```python
from build123d import *

# Parameters (mm, degrees)
BOSS_EXTRU_1_DEPTH      = 36
ESQUISSE2_W             = 34
ESQUISSE2_H             = 20
BOSS_EXTRU_2_DEPTH      = 2
ESQUISSE3_R             = 6
BOSS_EXTRU_3_DEPTH      = 2
ESQUISSE4_R             = 2.5
BOSS_EXTRU_4_DEPTH      = 4
ESQUISSE5_W             = 20
ESQUISSE5_H             = 2.5
BOSS_EXTRU_5_DEPTH      = 7
ENL_V_MAT_EXTRU_1_REACH = 53.585
ESQUISSE6_R             = 2
CONG_1_R                = 2
ESQUISSE7_W             = 20
ESQUISSE7_H             = 2.5
BOSS_EXTRU_6_DEPTH      = 7
ENL_V_MAT_EXTRU_2_REACH = 59.184
ESQUISSE8_R             = 2
CONG_2_R                = 2


with BuildPart() as part:
    # Esquisse1 → Boss.-Extru.1 (new body)
    with BuildSketch(Plane(origin=(0, 0, 0), x_dir=(1, 0, 0), z_dir=(0, 1, 0))):
        Polygon((0, 0), (0, 10), (40, 10), (40, -10), (0, -10), align=None)
    extrude(amount=BOSS_EXTRU_1_DEPTH)

    # Esquisse2 → Boss.-Extru.2 (add)
    with BuildSketch(Plane(origin=(0, 36, 0), x_dir=(1, 0, 0), z_dir=(0, 1, 0))):
        with Locations((23, 0)):
            Rectangle(ESQUISSE2_W, ESQUISSE2_H)
    extrude(amount=BOSS_EXTRU_2_DEPTH)

    # Esquisse3 → Boss.-Extru.3 (add)
    with BuildSketch(Plane(origin=(0, 38, 0), x_dir=(1, 0, 0), z_dir=(0, 1, 0))):
        with Locations(Location((32, 0, 0), (0, 0, 90))):
            Circle(ESQUISSE3_R)
    extrude(amount=BOSS_EXTRU_3_DEPTH)

    # Esquisse4 → Boss.-Extru.4 (add)
    with BuildSketch(Plane(origin=(0, 40, 0), x_dir=(1, 0, 0), z_dir=(0, 1, 0))):
        with Locations(Location((32, 0, 0), (0, 0, 270))):
            Circle(ESQUISSE4_R)
    extrude(amount=BOSS_EXTRU_4_DEPTH)

    # Esquisse5 → Boss.-Extru.5 (add)
    with BuildSketch(Plane.ZY):
        with Locations((0, 29.75)):
            Rectangle(ESQUISSE5_W, ESQUISSE5_H)
    extrude(amount=BOSS_EXTRU_5_DEPTH)

    # Esquisse6 → Enlèv. mat.-Extru.1 (cut, up to next)
    with BuildSketch(Plane(origin=(0, 31, 0), x_dir=(1, 0, 0), z_dir=(0, 1, 0)), mode=Mode.PRIVATE) as enl_v_mat_extru_1_sk1:
        with Locations(Location((-4.5, 5, 0), (0, 0, 270))):
            Circle(ESQUISSE6_R)
    enl_v_mat_extru_1_tool1 = extrude(enl_v_mat_extru_1_sk1.sketch, amount=-ENL_V_MAT_EXTRU_1_REACH, mode=Mode.PRIVATE) & part.part
    # Esquisse6 → Enlèv. mat.-Extru.1 (cut, up to next)
    with BuildSketch(Plane(origin=(0, 31, 0), x_dir=(1, 0, 0), z_dir=(0, 1, 0)), mode=Mode.PRIVATE) as enl_v_mat_extru_1_sk2:
        with Locations(Location((-4.5, -5, 0), (0, 0, 270))):
            Circle(ESQUISSE6_R)
    enl_v_mat_extru_1_tool2 = extrude(enl_v_mat_extru_1_sk2.sketch, amount=-ENL_V_MAT_EXTRU_1_REACH, mode=Mode.PRIVATE) & part.part
    add(enl_v_mat_extru_1_tool1.solids().sort_by_distance((-4.5, 31, -5))[0], mode=Mode.SUBTRACT)
    add(enl_v_mat_extru_1_tool2.solids().sort_by_distance((-4.5, 31, 5))[0], mode=Mode.SUBTRACT)

    # Congé1
    cong_1_edges = [part.edges().sort_by_distance(p)[0] for p in [
        (0, 14.25, 10),
        (0, 14.25, -10),
        (-7, 29.75, -10),
        (-7, 29.75, 10),
        (0, 33.5, -10),
        (0, 33.5, 10),
    ]]
    fillet(cong_1_edges, radius=CONG_1_R)

    # Esquisse7 → Boss.-Extru.6 (add)
    with BuildSketch(Plane(origin=(40, 0, 0), x_dir=(0, 0, -1), z_dir=(1, 0, 0))):
        with Locations((0, 29.75)):
            Rectangle(ESQUISSE7_W, ESQUISSE7_H)
    extrude(amount=BOSS_EXTRU_6_DEPTH)

    # Esquisse8 → Enlèv. mat.-Extru.2 (cut, up to next)
    with BuildSketch(Plane(origin=(0, 31, 0), x_dir=(1, 0, 0), z_dir=(0, 1, 0)), mode=Mode.PRIVATE) as enl_v_mat_extru_2_sk1:
        with Locations(Location((44.5, 5, 0), (0, 0, 270))):
            Circle(ESQUISSE8_R)
    enl_v_mat_extru_2_tool1 = extrude(enl_v_mat_extru_2_sk1.sketch, amount=-ENL_V_MAT_EXTRU_2_REACH, mode=Mode.PRIVATE) & part.part
    # Esquisse8 → Enlèv. mat.-Extru.2 (cut, up to next)
    with BuildSketch(Plane(origin=(0, 31, 0), x_dir=(1, 0, 0), z_dir=(0, 1, 0)), mode=Mode.PRIVATE) as enl_v_mat_extru_2_sk2:
        with Locations(Location((44.5, -5, 0), (0, 0, 270))):
            Circle(ESQUISSE8_R)
    enl_v_mat_extru_2_tool2 = extrude(enl_v_mat_extru_2_sk2.sketch, amount=-ENL_V_MAT_EXTRU_2_REACH, mode=Mode.PRIVATE) & part.part
    add(enl_v_mat_extru_2_tool1.solids().sort_by_distance((44.5, 31, -5))[0], mode=Mode.SUBTRACT)
    add(enl_v_mat_extru_2_tool2.solids().sort_by_distance((44.5, 31, 5))[0], mode=Mode.SUBTRACT)

    # Congé2
    cong_2_edges = [part.edges().sort_by_distance(p)[0] for p in [
        (40, 14.25, -10),
        (40, 14.25, 10),
        (47, 29.75, 10),
        (47, 29.75, -10),
        (40, 34.5, -10),
        (40, 34.5, 10),
    ]]
    fillet(cong_2_edges, radius=CONG_2_R)


solid = part.part
```
CAD build for the part. Positions are in the model's coordinates, mm. A direction names the side the tool comes from. Give positions to 0.01 mm unless a question says otherwise; leave off trailing zeros. Write each loop counter-clockwise with the first axis right and the second up, starting at its lowest first coordinate (ties: lowest second). Pieces come first, ordered by that corner, then holes. Notation, with made-up numbers: M 24.25,47 L 51.25,47 A33 ccw 51.25,75 Z; hole C 83,61.5 d10. An arc over 180 degrees is marked long. Return JSON: item names as keys, results as strings. Group by question number.
(1) 3-axis set-ups, long thin cutter, end or side, ignore diameter. For faces 1 (the face through (39.43, 34.45, -9.4)), 2 (the face through (0, 14, 0)), 3 (the face through (39.4, 34.55, 9.43)), 4 (the face through (37.857, 38.986, 1.301)): which of +Z, -Z, +X, -X, +Y, -Y reach the whole face in a straight line?
(2) Drill centre lines: L1, parallel to X at y = 30.15, z = -5; L2, parallel to Z at x = 44, y = 29; L3, parallel to Y at x = 33.5, z = 8.5. Where is each one in solid material? Low to high. Write a range as [from, to].
(3) Band-saw the part on A-A (y = 10). Give the cut face in (x, z), and give its area (3 significant figures).
(4) Band-saw the part on B-B (z = -5). Give the cut face in (x, y), and give its area (3 significant figures).
(5) Flat gauge pins, fed straight in: pin 1 Ø2.5 at (x, z) = (-4.5, -5) entering from +Y; pin 2 Ø1.5 at (y, z) = (33.5, 2.5) entering from -X; pin 3 Ø3 at (x, z) = (2, 0) entering from +Y; pin 4 Ø7.5 at (y, z) = (35, 3.5) entering from +X. Where does each tip first touch, or does it go through?
(6) Band-saw the part on D-D (z = 0). Give the cut face in (x, y).
(7) Band-saw the part on C-C (x = 32). Give the cut face in (y, z), and give its area (3 significant figures).
Entries:
{
 "1": {"face 1": "-Z, +X, +Y", "face 2": "+Z, -Z, -X, -Y", "face 3": "+Z, +X, +Y", "face 4": "+Y"},
 "2": {"L1": "x = [-7, -6.5], [-2.5, 42.5], [46.5, 47]", "L2": "z = [-10, -6.94], [-3.06, 3.06], [6.94, 10]", "L3": "y = [0, 38]"},
 "3": {"outline": "M 0,-8 A2 ccw 2,-10 L 38,-10 A2 ccw 40,-8 L 40,8 A2 ccw 38,10 L 2,10 A2 ccw 0,8 Z", "area": "797 mm^2"},
 "4": {"outline": "M -7,28.5 L -6.5,28.5 L -6.5,31 L -7,31 Z; M -2.5,28.5 L 0,28.5 L 0,0 L 40,0 L 40,28.5 L 42.5,28.5 L 42.5,31 L 40,31 L 40,38 L 35.32,38 L 35.32,40 L 28.68,40 L 28.68,38 L 6,38 L 6,36 L 0,36 L 0,31 L -2.5,31 Z; M 46.5,28.5 L 47,28.5 L 47,31 L 46.5,31 Z", "area": "1,540 mm^2"},
 "5": {"pin 1": "passes through", "pin 2": "stops at x = 0", "pin 3": "stops at y = 36", "pin 4": "stops at x = 40"},
 "6": {"outline": "M -7,28.5 L 0,28.5 L 0,0 L 40,0 L 40,28.5 L 47,28.5 L 47,31 L 40,31 L 40,38 L 38,38 L 38,40 L 34.5,40 L 34.5,44 L 29.5,44 L 29.5,40 L 26,40 L 26,38 L 6,38 L 6,36 L 0,36 L 0,31 L -7,31 Z"},
 "7": {"outline": "M 0,-10 L 38,-10 L 38,-6 L 40,-6 L 40,-2.5 L 44,-2.5 L 44,2.5 L 40,2.5 L 40,6 L 38,6 L 38,10 L 0,10 Z", "area": "804 mm^2"}
}
